```python
from build123d import *

# Parameters (mm, degrees)
F0_W     = 102.7466543019
F0_H     = 90.9466221929
F0_W_2   = 85.1905047894
F0_H_2   = 44.8976957705
F1_DEPTH = 152.4
F2_R     = 11.1763524663
F3_DEPTH = 76.2


with BuildPart() as f1:
    # F0 (on Front) → F1 (new body)
    with BuildSketch(Plane.XZ):
        with Locations((-1.8626e-06, 7.9146586359)):
            Rectangle(F0_W, F0_H)
        Polygon((-41.8757386506, -12.8073554952), (-41.8757386506, -7.9146586359), (-37.270847708, -7.9146586359), (-24.3195872754, -7.9146586359), (-24.3195872754, -18.5634717345), (-37.270847708, -18.5634717345), (-41.8757386506, -18.5634717345), align=None, mode=Mode.SUBTRACT)
        with BuildLine():
            Line((-15.3976082802, -30.6513141841), (-15.3976082802, -23.7439740449))
            Line((-15.3976082802, -23.7439740449), (25.5187885163, -23.7439740449))
            Line((25.5187885163, -23.7439740449), (25.5187885163, -30.6513141841))
            Line((25.5187885163, -30.6513141841), (23.2219085714, -30.6513141841))
            add(Edge.make_bspline(
                [(23.2219085714, -30.6513141841), (22.85194256, -30.745750475), (22.4083868695, -30.745750475)],
                knots=[0.6101406025, 0.6101406025, 0.6101406025, 1, 1, 1], degree=2))
            add(Edge.make_bspline(
                [(22.4083868695, -30.745750475), (21.9525027452, -30.745750475), (21.5799819799, -30.6513141841)],
                knots=[0, 0, 0, 0.4594075276, 0.4594075276, 0.4594075276], degree=2))
            Line((21.5799819799, -30.6513141841), (17.1949040127, -30.6513141841))
            Line((17.1949040127, -30.6513141841), (15.8233293106, -30.6513141841))
            Line((15.8233293106, -30.6513141841), (12.6383256981, -30.6513141841))
            add(Edge.make_bspline(
                [(12.6383256981, -30.6513141841), (12.2965846392, -30.745750475), (11.8839868875, -30.745750475)],
                knots=[0.6033851102, 0.6033851102, 0.6033851102, 1, 1, 1], degree=2))
            add(Edge.make_bspline(
                [(11.8839868875, -30.745750475), (11.4876624367, -30.745750475), (11.1537473039, -30.6513141841)],
                knots=[0, 0, 0, 0.3398387497, 0.3398387497, 0.3398387497], degree=2))
            Line((11.1537473039, -30.6513141841), (3.1983305145, -30.6513141841))
            add(Edge.make_bspline(
                [(3.1983305145, -30.6513141841), (2.7104556951, -30.745750475), (2.1975216142, -30.745750475)],
                knots=[0.4435987872, 0.4435987872, 0.4435987872, 1, 1, 1], degree=2))
            add(Edge.make_bspline(
                [(2.1975216142, -30.745750475), (1.6733949816, -30.745750475), (1.2280841955, -30.6513141841)],
                knots=[0, 0, 0, 0.325259052, 0.325259052, 0.325259052], degree=2))
            Line((1.2280841955, -30.6513141841), (-2.1870204663, -30.6513141841))
            Line((-2.1870204663, -30.6513141841), (-3.5690880896, -30.6513141841))
            Line((-3.5690880896, -30.6513141841), (-6.4456474922, -30.6513141841))
            Line((-6.4456474922, -30.6513141841), (-7.8277151155, -30.6513141841))
            Line((-7.8277151155, -30.6513141841), (-11.0580714674, -30.6513141841))
            add(Edge.make_bspline(
                [(-11.0580714674, -30.6513141841), (-11.4916109594, -30.745750475), (-12.0113927042, -30.745750475)],
                knots=[0.6303252294, 0.6303252294, 0.6303252294, 1, 1, 1], degree=2))
            add(Edge.make_bspline(
                [(-12.0113927042, -30.745750475), (-12.5246569888, -30.745750475), (-12.9473134807, -30.6513141841)],
                knots=[0, 0, 0, 0.3766854018, 0.3766854018, 0.3766854018], degree=2))
            Line((-12.9473134807, -30.6513141841), (-15.3976082802, -30.6513141841))
        make_face(mode=Mode.SUBTRACT)
        Polygon((14.5341921598, -17.9878585041), (14.5341921598, -7.6268524863), (26.0464195162, -7.6268524863), (31.5147265792, -7.6268524863), (31.5147265792, -12.8073554952), (31.5147265792, -17.9878585041), (26.0464195162, -17.9878585041), align=None, mode=Mode.SUBTRACT)
        with Locations((1.2951269746, 25.7586139487)):
            Rectangle(F0_W_2, F0_H_2, mode=Mode.SUBTRACT)
    extrude(amount=F1_DEPTH)

    # F2 (on Right) → F3 (join)
    with BuildSketch(Plane.YZ):
        with Locations((-8.1405537203, -48.4952703118)):
            Circle(F2_R)
        with BuildLine():
            ThreePointArc((-144.905696857, -39.7735155561), (-145.56909186, -58.572575633), (-129.1690343005, -49.3593859167))
            ThreePointArc((-129.1690343005, -49.3593859167), (-130.8108710033, -43.6385160791), (-135.2366314328, -39.6589904693))
            ThreePointArc((-135.2366314328, -39.6589904693), (-140.084714499, -38.57223065), (-144.905696857, -39.7735155561))
        make_face()
        with BuildLine():
            ThreePointArc((-144.905696857, -39.7735155561), (-140.084714499, -38.57223065), (-135.2366314328, -39.6589904693))
            Line((-135.2366314328, -39.6589904693), (-135.2366314328, -34.9684022367))
            Line((-135.2366314328, -34.9684022367), (-142.5458490849, -34.9684022367))
            Line((-142.5458490849, -34.9684022367), (-144.905696857, -39.7735155561))
        make_face()
    extrude(amount=F3_DEPTH)


solid = f1.part
```
Verification items for the finished model (mm, model axes). A direction names the side the tool comes from. Coordinates: 2 decimals unless noted, no trailing zeros. Write each loop counter-clockwise with the first axis right and the second up, starting at its lowest first coordinate (ties: lowest second). Pieces come first, ordered by that corner, then holes. Notation, with made-up numbers: M -13.75,62.5 L 4.25,62.5 A27 cw 4.25,87.5 Z; hole C 36.25,3 d4. An arc over 180 degrees is marked long. One line per item, written item: value.
Item 1: Section check A-A, the plane z = -11. Record the boundary of the cut face in (x, y), plus the area to 3 significant figures.
Check sheet entries:
outline: M -51.37,-152.4 L -41.88,-152.4 L -41.88,0 L -51.37,0 Z; M -24.32,-152.4 L 14.53,-152.4 L 14.53,0 L -24.32,0 Z; M 31.51,-152.4 L 51.37,-152.4 L 51.37,0 L 31.51,0 Z
area: 10,400 mm^2
Item 2: Section check B-B, the plane z = 29. Record the boundary of the cut face in (x, y).
Check sheet entries:
outline: M -51.37,-152.4 L -41.3,-152.4 L -41.3,0 L -51.37,0 Z; M 43.89,-152.4 L 51.37,-152.4 L 51.37,0 L 43.89,0 Z
Item 3: Gauge pin test, flat ends, axial feed: pin 1 Ø3 at (y, z) = (-96, 25) entering from +X; pin 2 Ø6.5 at (y, z) = (-145, -45.5) entering from -X; pin 3 Ø19.5 at (x, y) = (-36, -70) entering from -Z. Record the tip position at first contact, or that the pin passes through.
Check sheet entries:
pin 1: stops at x = 51.37
pin 2: stops at x = 0
pin 3: stops at z = -37.56
Item 4: Section check D-D, the plane y = -132.5. State how many separate pieces and enclosed holes the cut face has, plus the area to 3 significant figures.
Check sheet entries:
separate pieces: 2
enclosed holes: 4
area: 6,060 mm^2
Item 5: Scan lines: line 1 along Z through (x, y) = (9.5, -121); line 2 along Z through (x, y) = (26, -48); line 3 along X through (y, z) = (-99, 29.5). Record each from-to range of solid material in increasing order.
Check sheet entries:
line 1: z = -37.56 to -30.65, -23.74 to 3.31, 48.21 to 53.39
line 2: z = -37.56 to -17.99, -7.63 to 3.31, 48.21 to 53.39
line 3: x = -51.37 to -41.3, 43.89 to 51.37
Item 6: Section check C-C, the plane x = 17. Record the boundary of the cut face in (y, z).
Check sheet entries:
outline: M -152.4,-37.56 L -143.82,-37.56 L -144.91,-39.77 A10.79 ccw long -135.24,-39.66 L -135.24,-37.56 L -10.44,-37.56 A11.18 ccw long -5.84,-37.56 L 0,-37.56 L 0,-30.65 L -152.4,-30.65 Z; M -152.4,-23.74 L 0,-23.74 L 0,-17.99 L -152.4,-17.99 Z; M -152.4,-7.63 L 0,-7.63 L 0,3.31 L -152.4,3.31 Z; M -152.4,48.21 L 0,48.21 L 0,53.39 L -152.4,53.39 Z
Item 7: Access from +Z, -Z, +X, -X, +Y, -Y to the whole of each face (thin tool, end or side, straight path). Record for faces 4 (the flat face through (-1, 0, -2)), 5 (the flat face through (-15.398, -75, -27)), 6 (the flat face through (0, -8, -48)).
Check sheet entries:
face 4: +Z, +X, -X, +Y
face 5: +Y, -Y
face 6: -Z, -X, +Y, -Y
Item 8: Mould release check, pull along Z, two halves, no side actions. Record for faces 1 (the flat face through (-5, -75, -30.651)), 2 (the flat face through (-1, -152.4, -2)), 3 (the flat face through (-24.32, -75, -13)): pulls with the +Z half, pulls with the -Z half, needs draft (parallel to the pull), parting line crosses it, or undercut.
Check sheet entries:
face 1: undercut
face 2: needs draft
face 3: undercut
